Work out the finished part from the listing and answer in its coordinate system (mm). Face numbers are marked on the shaded views. A direction names the side the tool comes from. Round coordinates to 2 decimals unless told otherwise and drop trailing zeros. Order: outer loops, then holes, each group sorted by start corner. A loop starts at its lowest first (then second) coordinate and runs counter-clockwise, first axis right, second up. Notation, with made-up numbers: (-39.75, 69.5) - (-28.75, 69.5) arc R16 cw to (-28.75, 82.5) - close; hole circle Ø6 at (10, -32). An arc over 180 degrees is marked (long way). Use CSV: the item, a comma, the result in double quotes.
from build123d import *

# Parameters (mm, degrees)
SKETCH1_R                = 45.72
SKETCH1_R_2              = 38.1
BOSS_EXTRUDE1_DEPTH      = 20.32
BOSS_EXTRUDE1_DEPTH_BACK = 20.32
SKETCH1_4_R              = 20.0025
BOSS_EXTRUDE2_DEPTH      = 43.18
BOSS_EXTRUDE2_DEPTH_BACK = 55.88
CHAMFER1_SIZE            = 17.62
FILLET1_R                = 17.62
BOSS_EXTRUDE3_DEPTH      = 3.175
BOSS_EXTRUDE4_DEPTH      = 3.175
SKETCH4_W                = 19.05
SKETCH4_H                = 40.64
BOSS_EXTRUDE5_DEPTH      = 3.175


with BuildPart() as part:
    # Sketch1 → Boss-Extrude1 (new body, two sides)
    with BuildSketch(Plane(origin=(0, 0, 0), x_dir=(1, 0, 0), z_dir=(0, 1, 0))) as boss_extrude1_sk:
        Circle(SKETCH1_R)
        Circle(SKETCH1_R_2, mode=Mode.SUBTRACT)
    extrude(amount=BOSS_EXTRUDE1_DEPTH)
    extrude(boss_extrude1_sk.sketch, amount=-BOSS_EXTRUDE1_DEPTH_BACK)



with BuildPart() as body_2:
    # Sketch1_4 → Boss-Extrude2 (new body, two sides)
    with BuildSketch(Plane(origin=(0, 0, 0), x_dir=(1, 0, 0), z_dir=(0, 1, 0))) as boss_extrude2_sk:
        Circle(SKETCH1_4_R)
    extrude(amount=BOSS_EXTRUDE2_DEPTH)
    extrude(boss_extrude2_sk.sketch, amount=-BOSS_EXTRUDE2_DEPTH_BACK)

    # Chamfer1
    chamfer1_edges = [body_2.edges().sort_by_distance(p)[0] for p in [
        (-20.0025, -55.88, 0),
    ]]
    chamfer(chamfer1_edges, length=CHAMFER1_SIZE)

    # Fillet1
    fillet1_edges = [body_2.edges().sort_by_distance(p)[0] for p in [
        (-20.0025, 43.18, 0),
    ]]
    fillet(fillet1_edges, radius=FILLET1_R)

    # Sketch2 → Boss-Extrude3 (add)
    with BuildSketch(Plane(origin=(0, 0, 0), x_dir=(1, 0, 0), z_dir=(0, 1, 0))):
        Polygon((17.58904151, 9.525), (35.36904151, 6.389906283), (35.36904151, -6.389906283), (17.58904151, -9.525), (17.58904151, 0), align=None)
        Polygon((-23.218341924, -27.435535314), (-17.043412726, -10.470056776), (-8.794520755, -15.232556776), (-0.545628784, -19.995056776), (-12.150699586, -33.825441597), align=None)
        Polygon((-12.150699586, 33.825441597), (-0.545628784, 19.995056776), (-8.794520755, 15.232556776), (-17.043412726, 10.470056776), (-23.218341924, 27.435535314), align=None)
    extrude(amount=BOSS_EXTRUDE3_DEPTH)


with BuildPart() as part_1:
    add(part.part)

    add(body_2.part)  # Boss-Extrude4 merges body 2
    # Sketch3 → Boss-Extrude4 (add)
    with BuildSketch(Plane.XZ.offset(20.32)):
        with BuildLine():
            ThreePointArc((38.1, -2.54), (40.64, 0), (38.1, 2.54))
            Line((38.1, 2.54), (2.54, 2.54))
            Line((2.54, 2.54), (2.54, -2.54))
            Line((2.54, -2.54), (38.1, -2.54))
        make_face()
        with BuildLine():
            Line((-2.54, 2.54), (2.54, 2.54))
            Line((2.54, 2.54), (2.54, 38.1))
            ThreePointArc((2.54, 38.1), (0, 40.64), (-2.54, 38.1))
            Line((-2.54, 38.1), (-2.54, 2.54))
        make_face()
        with BuildLine():
            Line((2.54, -38.1), (2.54, -2.54))
            Line((2.54, -2.54), (-2.54, -2.54))
            Line((-2.54, -2.54), (-2.54, -38.1))
            ThreePointArc((-2.54, -38.1), (0, -40.64), (2.54, -38.1))
        make_face()
        with BuildLine():
            Line((-2.54, -2.54), (-2.54, 2.54))
            Line((-2.54, 2.54), (-38.1, 2.54))
            ThreePointArc((-38.1, 2.54), (-40.64, 0), (-38.1, -2.54))
            Line((-38.1, -2.54), (-2.54, -2.54))
        make_face()
    extrude(amount=-BOSS_EXTRUDE4_DEPTH)

    # Sketch4 → Boss-Extrude5 (add)
    with BuildSketch(Plane(origin=(0, 0, -45.72), x_dir=(-1, 0, 0), z_dir=(0, 0, -1))):
        Rectangle(SKETCH4_W, SKETCH4_H)
    extrude(amount=-BOSS_EXTRUDE5_DEPTH)


solid = part_1.part
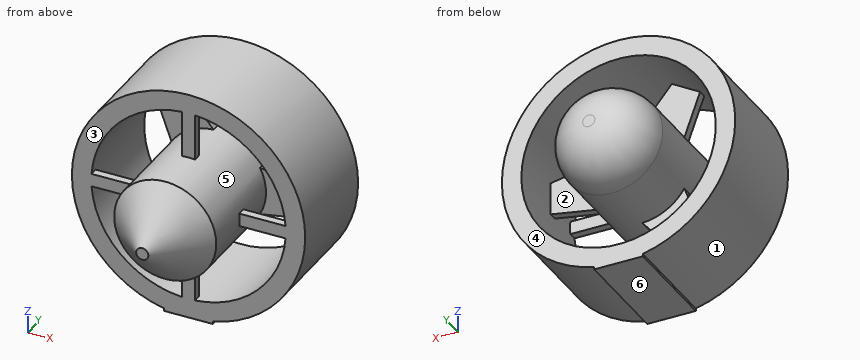
(1) For the marked faces 4, 5 and 6, determine the directions among +Z, -Z, +X, -X, +Y, -Y from which every point of the face is accessible in a straight line to the end or side of a thin tool.
Findings below:
face 4,"+Y"
face 5,"none"
face 6,"-Z, +X, -X, +Y, -Y"
(2) Find section D-D (y = -32). Determine the outline of the cut face in (x, z) (1 decimal).
Findings below:
outline,"circle Ø40 at (0, 0)"
(3) Find section B-B (z = 29.5). Determine the outline of the cut face in (x, y) (3 decimals).
Findings below:
outline,"(-34.929, -20.32) - (-24.111, -20.32) - (-24.111, 20.32) - (-34.929, 20.32) - close; (-19.643, 0) - (-8.521, 0) - (-8.521, 3.175) - (-19.643, 3.175) - close; (-2.54, -20.32) - (2.54, -20.32) - (2.54, -17.145) - (-2.54, -17.145) - close; (24.111, -20.32) - (34.929, -20.32) - (34.929, 20.32) - (24.111, 20.32) - close"
(4) Each of these flat-tipped pins is pushed along its axis until it touches: pin 1 (1.5 mm diameter, centred on x = 24, z = -4.5, fed in from +Y) (3 decimals); pin 2 (12 mm diameter, centred on x = 7.5, y = -4.5, fed in from +Z); pin 3 (4 mm diameter, centred on y = -42, z = -11.5, fed in from +X). Where does it stop, or does it pass through?
Findings below:
pin 1,"stops at y = 3.175"
pin 2,"stops at z = 45.7"
pin 3,"stops at x = 14.61"
(5) Find the intervals of material crossed by L1, parallel to X at y = 8, z = 0; L2, parallel to Z at x = 2, y = 18; L3, parallel to X at y = 14.5, z = -14, in increasing order. Write a range as from..to.
Findings below:
L1,"x = -45.72..-38.1, -20..20, 38.1..45.72"
L2,"z = -45.72..-38.05, -19.9..19.9, 38.05..45.68"
L3,"x = -43.52..-35.43, -14.29..14.29, 35.43..43.52"
(6) Find section C-C (z = -4). State how many separate pieces and enclosed holes the cut face has, and give its area (3 significant figures).
Findings below:
separate pieces,"3"
enclosed holes,"0"
area,"4,080 mm²"
(7) The mould has two halves that part along X. Classify the marked faces 1, 2 and 3: released by +X, released by -X, zero draft, split by the parting line, or undercut.
Findings below:
face 1,"split by the parting line"
face 2,"undercut"
face 3,"zero draft"
(8) Find section A-A (x = 33.5). Determine the outline of the cut face in (y, z) (3 decimals), and give its area (3 significant figures).
Findings below:
outline,"(-20.32, -31.114) - (20.32, -31.114) - (20.32, -18.148) - (-20.32, -18.148) - close; (-20.32, -2.54) - (-17.145, -2.54) - (-17.145, 2.54) - (-20.32, 2.54) - close; (-20.32, 18.148) - (20.32, 18.148) - (20.32, 31.114) - (-20.32, 31.114) - close; (0, -6.719) - (3.175, -6.719) - (3.175, 6.719) - (0, 6.719) - close"
area,"1,110 mm²"
